```python
from build123d import *

# Parameters (mm, degrees)
CHAMFER1_SIZE = 0.5
FILLET1_R     = 0.2


with BuildPart() as part:
    # Sketch2 → Revolve1 (revolve)
    with BuildSketch(Plane.XY):
        Polygon((0, 0), (0, 25), (4, 25), (4, 23), (0.9, 23), (0.9, 20.5), (2, 20.5), (2, 18.5), (1, 18.5), (1, 0), align=None)
    revolve(axis=Axis((0, 0, 0), (0, 1, 0)))

    # Chamfer1
    chamfer1_edges = [part.edges().sort_by_distance(p)[0] for p in [
        (-2, 20.5, 0),
    ]]
    chamfer(chamfer1_edges, length=CHAMFER1_SIZE)

    # Fillet1
    fillet1_edges = [part.edges().sort_by_distance(p)[0] for p in [
        (-0.9, 23, 0),
        (-1, 18.5, 0),
        (-0.9, 20.5, 0),
    ]]
    fillet(fillet1_edges, radius=FILLET1_R)


solid = part.part
```
The listing builds one solid part. Answer for the finished solid, in the listing's coordinates (mm). A direction names the side the tool comes from. Round coordinates to 2 decimals unless told otherwise and drop trailing zeros. Write each loop counter-clockwise with the first axis right and the second up, starting at its lowest first coordinate (ties: lowest second). Pieces come first, ordered by that corner, then holes. Notation, with made-up numbers: (-34, 73) -> (-29, 73) arc R22 cw to (-29, 94) -> close; hole circle Ø5 at (-4, -14). An arc over 180 degrees is marked (long way). Use CSV: the item, a comma, the result in double quotes. Start each with the question number.
(1) Each of these flat-tipped pins is pushed along its axis until it touches: pin 1 (3 mm diameter, centred on x = 3, y = 15.5, fed in from -Z); pin 2 (1 mm diameter, centred on x = 3, z = -2, fed in from -Y). Where does it stop, or does it pass through?
(2) Section D-D on x = 3.75 is taken. Give the vertices of the cut face in (y, z), then the cut area to 3 significant figures.
(3) Which of the six approach directions +Z, -Z, +X, -X, +Y, -Y give full straight-line access (tool end or side, diameter ignored) to faces 1 (the face through (0, 9, 1)), 2 (the face through (-0.867, 23.986, 3.905)), 3 (the face through (1, 23, 1))?
(4) Consider L1, parallel to Y at x = -1, z = 2.25; L2, parallel to X at y = 5.25, z = 0; L3, parallel to Y at x = 0.25, z = -1.5. Determine where each line is inside the solid, lowest interval first. Write a range as from..to.
(5) Section C-C on z = -3.25 is taken. Give the vertices of the cut face in (x, y), then the cut area to 3 significant figures.
(6) Section A-A on x = 0 is taken. Give the vertices of the cut face in (y, z).
(7) Section B-B on z = 0 is taken. Give the vertices of the cut face in (x, y).
(8) The mould has two halves that part along Y. Classify faces 4 (the face through (0, 19, 2)), 5 (the face through (0, 25, 0)), 6 (the face through (0.86, 21.74, -0.27)): released by +Y, released by -Y, zero draft, split by the parting line, or undercut.
A:
1,pin 1,"passes through"
1,pin 2,"stops at y = 23"
2,outline,"(23, -1.39) -> (25, -1.39) -> (25, 1.39) -> (23, 1.39) -> close"
2,area,"5.57 mm²"
3,face 1,"-Y"
3,face 2,"+Y, -Y"
3,face 3,"none"
4,L1,"y = 23..25"
4,L2,"x = -1..1"
4,L3,"y = 18.5..20.48, 23..25"
5,outline,"(-2.33, 23) -> (2.33, 23) -> (2.33, 25) -> (-2.33, 25) -> close"
5,area,"9.33 mm²"
6,outline,"(0, -1) -> (18.3, -1) arc R0.2 cw to (18.5, -1.2) -> (18.5, -2) -> (20, -2) -> (20.5, -1.5) -> (20.5, -1.1) arc R0.2 cw to (20.7, -0.9) -> (22.8, -0.9) arc R0.2 cw to (23, -1.1) -> (23, -4) -> (25, -4) -> (25, 4) -> (23, 4) -> (23, 1.1) arc R0.2 cw to (22.8, 0.9) -> (20.7, 0.9) arc R0.2 cw to (20.5, 1.1) -> (20.5, 1.5) -> (20, 2) -> (18.5, 2) -> (18.5, 1.2) arc R0.2 cw to (18.3, 1) -> (0, 1) -> close"
7,outline,"(-4, 23) -> (-1.1, 23) arc R0.2 cw to (-0.9, 22.8) -> (-0.9, 20.7) arc R0.2 cw to (-1.1, 20.5) -> (-1.5, 20.5) -> (-2, 20) -> (-2, 18.5) -> (-1.2, 18.5) arc R0.2 cw to (-1, 18.3) -> (-1, 0) -> (1, 0) -> (1, 18.3) arc R0.2 cw to (1.2, 18.5) -> (2, 18.5) -> (2, 20) -> (1.5, 20.5) -> (1.1, 20.5) arc R0.2 cw to (0.9, 20.7) -> (0.9, 22.8) arc R0.2 cw to (1.1, 23) -> (4, 23) -> (4, 25) -> (-4, 25) -> close"
8,face 4,"zero draft"
8,face 5,"released by +Y"
8,face 6,"undercut"
